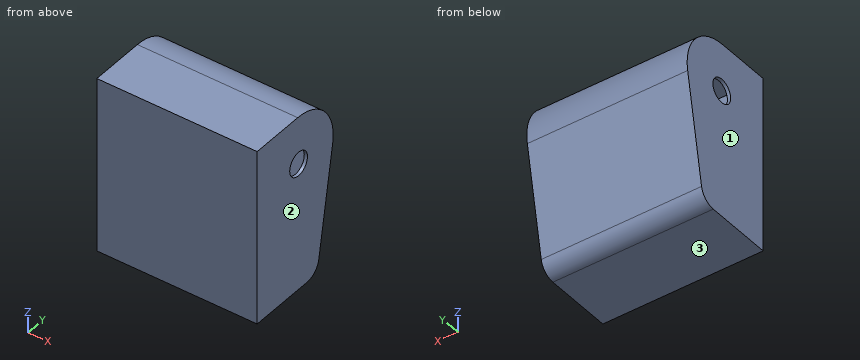
from build123d import *

# Parameters (mm, degrees)
SKETCH_271_W          = 1100
SKETCH_271_H          = 700
EXTRUDE_334_DEPTH     = 1000
DRAFT_385_ANGLE       = -10
FILLET_1_R            = 300
FILLET_2_R            = 100
SHELL_626_T           = 20
SKETCH_649_R          = 75
CUT_EXTRUDE_760_DEPTH = 1620.497681608


with BuildPart() as part:
    # Sketch 271 → Extrude 334 (new body)
    with BuildSketch(Plane(origin=(0, 0, 0), x_dir=(0, 0, -1), z_dir=(1, 0, 0))):
        with Locations((550, 350)):
            Rectangle(SKETCH_271_W, SKETCH_271_H)
    extrude(amount=EXTRUDE_334_DEPTH)

    # Draft 385
    draft_385_faces = [part.faces().sort_by_distance(p)[0] for p in [
        (500, 700, -550),
    ]]
    draft(draft_385_faces, Plane(origin=(1000, 0, 0), x_dir=(1, 0, 0), z_dir=(0, 0, 1)), DRAFT_385_ANGLE)

    # Скруглення1
    fillet_1_edges = [part.edges().sort_by_distance(p)[0] for p in [
        (500, 700, 0),
    ]]
    fillet(fillet_1_edges, radius=FILLET_1_R)

    # Скруглення2
    fillet_2_edges = [part.edges().sort_by_distance(p)[0] for p in [
        (500, 506.040321221, -1100),
    ]]
    fillet(fillet_2_edges, radius=FILLET_2_R)

    # Shell 626 (no face opened: a closed hollow body)
    add(offset(amount=-SHELL_626_T, mode=Mode.PRIVATE), mode=Mode.SUBTRACT)

    # Sketch 649 → Cut-Extrude 760 (cut, through all)
    with BuildSketch(Plane(origin=(0, 0, 0), x_dir=(0, 0, -1), z_dir=(1, 0, 0))):
        with Locations(Location((300, 350, 0), (0, 0, 180))):
            Circle(SKETCH_649_R)
    extrude(amount=CUT_EXTRUDE_760_DEPTH, mode=Mode.SUBTRACT)


solid = part.part
Read the model definition and answer for the solid it produces. Units are mm, in the model's axes. Face numbers are marked on the shaded views. Give positions to 0.01 mm unless a question says otherwise; leave off trailing zeros. Write each loop counter-clockwise with the first axis right and the second up, starting at its lowest first coordinate (ties: lowest second). Pieces come first, ordered by that corner, then holes. Notation, with made-up numbers: (68.25, -3.5) -> (82.25, -3.5) arc R22 cw to (82.25, 28.5) -> close; hole circle Ø9 at (83, 9). An arc over 180 degrees is marked (long way). Answer as a JSON object with one key per item and string values. Group by question number.
1) The mould has two halves that part along X. Classify the marked faces 1, 2 and 3: +X half, -X half, draft (parallel to the pull), parting line (faces both ways), or undercut.
2) Consider L1, parallel to Z at x = 9.75, y = 350; L2, parallel to X at y = 426, z = -617; L3, parallel to Y at x = 995.75, z = -300. Determine where each line is inside the solid, lowest interval first. Write a range as from..to.
3) Find section C-C (z = -643). Write down the section's boundary in (x, y), and give its area (3 significant figures).
4) Find section D-D (z = -76.5). Write down the section's boundary in (x, y), and give its area (3 significant figures).
5) Find section B-B (x = 71). Write down the section's boundary in (y, z), and give its area (3 significant figures).
6) Find section A-A (z = -280.5). Write down the section's boundary in (x, y), and give its area (3 significant figures).
Values follow:
{
 "1": {"face 1": "-X half", "face 2": "+X half", "face 3": "draft"},
 "2": {"L1": "z = -1100..-375, -225..-0.09", "L2": "x = 0..20, 980..1000", "L3": "y = 0..275, 425..642.47"},
 "3": {"outline": "(0, 0) -> (1000, 0) -> (1000, 586.62) -> (0, 586.62) -> close; hole (20, 20) -> (980, 20) -> (980, 566.31) -> (20, 566.31) -> close", "area": "62,200 mm2"},
 "4": {"outline": "(0, 0) -> (1000, 0) -> (1000, 542.59) -> (0, 542.59) -> close; hole (20, 20) -> (980, 20) -> (980, 511.14) -> (20, 511.14) -> close", "area": "71,100 mm2"},
 "5": {"outline": "(0, -1100) -> (422.13, -1100) arc R100 ccw to (520.61, -1017.36) -> (637.92, -352.09) arc R300 ccw to (342.47, 0) -> (0, 0) -> close; hole (20, -1080) -> (422.13, -1080) arc R80 ccw to (500.91, -1013.89) -> (618.22, -348.62) arc R280 ccw to (342.47, -20) -> (20, -20) -> close", "area": "62,600 mm2"},
 "6": {"outline": "(0, 0) -> (1000, 0) -> (1000, 277.58) -> (980, 277.58) -> (980, 20) -> (20, 20) -> (20, 277.58) -> (0, 277.58) -> close; (0, 422.42) -> (20, 422.42) -> (20, 621.79) -> (980, 621.79) -> (980, 422.42) -> (1000, 422.42) -> (1000, 641.84) -> (0, 641.84) -> close", "area": "58,300 mm2"}
}
